Read the model definition and answer for the solid it produces. Units are mm, in the model's axes. Round coordinates to 2 decimals unless told otherwise and drop trailing zeros. Order: outer loops, then holes, each group sorted by start corner. A loop starts at its lowest first (then second) coordinate and runs counter-clockwise, first axis right, second up.
from build123d import *

# Parameters (mm, degrees)
SKETCH1_W           = 96
SKETCH1_H           = 128
BOSS_EXTRUDE1_DEPTH = 2.5
SKETCH2_R           = 1.6
CUT_EXTRUDE1_DEPTH  = 161.019530058
SKETCH3_R           = 1.6
CUT_EXTRUDE2_DEPTH  = 161.019530058
SKETCH4_R           = 1.5
CUT_EXTRUDE3_DEPTH  = 161.019530058
SKETCH9_R           = 1.6
CUT_EXTRUDE4_DEPTH  = 161.019530058
SKETCH12_R          = 3.5
CUT_EXTRUDE5_DEPTH  = 161.019530058
SKETCH13_W          = 23
SKETCH13_H          = 37
SKETCH13_W_2        = 26.25
SKETCH13_H_2        = 57.5
CUT_EXTRUDE6_DEPTH  = 161.019530058


with BuildPart() as part:
    # Sketch1 → Boss-Extrude1 (new body)
    with BuildSketch(Plane.XY):
        with Locations((48, 64)):
            Rectangle(SKETCH1_W, SKETCH1_H)
    extrude(amount=BOSS_EXTRUDE1_DEPTH)

    # Sketch2 → Cut-Extrude1 (cut, through all)
    with BuildSketch(Plane.XY.offset(2.5)):
        with Locations((2, 125)):
            Circle(SKETCH2_R)
        with Locations((27.4, 125)):
            Circle(SKETCH2_R)
        with Locations((78.47, 3)):
            Circle(SKETCH2_R)
        with Locations((68.39, 3)):
            Circle(SKETCH2_R)
        with BuildLine():
            Line((6.15, 126.65), (8.75, 126.65))
            ThreePointArc((8.75, 126.65), (10.4, 125), (8.75, 123.35))
            Line((8.75, 123.35), (6.15, 123.35))
            ThreePointArc((6.15, 123.35), (4.5, 125), (6.15, 126.65))
        make_face()
        with BuildLine():
            Line((87.25, 4.65), (89.85, 4.65))
            ThreePointArc((89.85, 4.65), (91.5, 3), (89.85, 1.35))
            Line((89.85, 1.35), (87.25, 1.35))
            ThreePointArc((87.25, 1.35), (85.6, 3), (87.25, 4.65))
        make_face()
    extrude(amount=-CUT_EXTRUDE1_DEPTH, mode=Mode.SUBTRACT)

    # Sketch3 → Cut-Extrude2 (cut, through all)
    with BuildSketch(Plane.XY.offset(2.5)):
        with Locations((25, 98)):
            Circle(SKETCH3_R)
        with Locations((60, 113)):
            Circle(SKETCH3_R)
        with Locations((25, 29.5)):
            Circle(SKETCH3_R)
    extrude(amount=-CUT_EXTRUDE2_DEPTH, mode=Mode.SUBTRACT)

    # Sketch4 → Cut-Extrude3 (cut, through all)
    with BuildSketch(Plane.XY.offset(2.5)):
        with Locations((13, 15)):
            Circle(SKETCH4_R)
        with Locations((63, 15)):
            Circle(SKETCH4_R)
    extrude(amount=-CUT_EXTRUDE3_DEPTH, mode=Mode.SUBTRACT)

    # Sketch9 → Cut-Extrude4 (cut, through all)
    with BuildSketch(Plane.XY.offset(2.5)):
        with Locations((9, 110.25)):
            Circle(SKETCH9_R)
        with Locations((9, 23.25)):
            Circle(SKETCH9_R)
        with Locations((86, 23.25)):
            Circle(SKETCH9_R)
        with Locations((86, 110.25)):
            Circle(SKETCH9_R)
    extrude(amount=-CUT_EXTRUDE4_DEPTH, mode=Mode.SUBTRACT)

    # Sketch12 → Cut-Extrude5 (cut, through all)
    with BuildSketch(Plane.XY.offset(2.5)):
        with Locations((16.73, 108.25)):
            Circle(SKETCH12_R)
        with Locations((16.73, 93.25)):
            Circle(SKETCH12_R)
        with Locations((16.73, 78.25)):
            Circle(SKETCH12_R)
        with Locations((16.73, 63.25)):
            Circle(SKETCH12_R)
        with Locations((16.73, 48.25)):
            Circle(SKETCH12_R)
        with Locations((16.73, 33.25)):
            Circle(SKETCH12_R)
        with Locations((60, 106.25)):
            Circle(SKETCH12_R)
        with Locations((60, 88.25)):
            Circle(SKETCH12_R)
        with Locations((60, 97.25)):
            Circle(SKETCH12_R)
        with Locations((84.5, 32)):
            Circle(SKETCH12_R)
        with Locations((84.5, 47)):
            Circle(SKETCH12_R)
    extrude(amount=-CUT_EXTRUDE5_DEPTH, mode=Mode.SUBTRACT)

    # Sketch13 → Cut-Extrude6 (cut, through all)
    with BuildSketch(Plane.XY.offset(2.5)):
        with Locations((80.5, 75.75)):
            Rectangle(SKETCH13_W, SKETCH13_H)
        with Locations((46.125, 51.25)):
            Rectangle(SKETCH13_W_2, SKETCH13_H_2)
    extrude(amount=-CUT_EXTRUDE6_DEPTH, mode=Mode.SUBTRACT)


solid = part.part
Q1. A cutting plane is placed at D-D, the plane y = 63.25. Give the vertices of the cut face in (x, z), plus the area to 3 significant figures.
Outcome:
outline: (0, 0) - (13.23, 0) - (13.23, 2.5) - (0, 2.5) - close; (20.23, 0) - (33, 0) - (33, 2.5) - (20.23, 2.5) - close; (59.25, 0) - (69, 0) - (69, 2.5) - (59.25, 2.5) - close; (92, 0) - (96, 0) - (96, 2.5) - (92, 2.5) - close
area: 99.4 mm2
Q2. A flat-ended cylindrical pin translates along its axis: pin 1 (0.8 mm diameter, centred on y = 83, z = 2, fed in from -X). Find the tip coordinate at first contact, or state that the pin passes through.
Outcome:
pin 1: stops at x = 0
Q3. A cutting plane is placed at C-C, the plane x = 38. Give the vertices of the cut face in (y, z), plus the area to 3 significant figures.
Outcome:
outline: (0, 0) - (22.5, 0) - (22.5, 2.5) - (0, 2.5) - close; (80, 0) - (128, 0) - (128, 2.5) - (80, 2.5) - close
area: 176 mm2
Q4. For a pull along X with two mould halves and no side action, classify faces 1 (the face through (96, 63, 1)), 2 (the face through (24.792, 99.586, 1.268)), 3 (the face through (84.4, 110.3, 1.3)), 4 (the face through (47, 0, 1)) as released by +X, released by -X, zero draft, split by the parting line, or undercut.
Outcome:
face 1: released by +X
face 2: undercut
face 3: undercut
face 4: zero draft
Q5. A cutting plane is placed at B-B, the plane x = 78.47. Give the vertices of the cut face in (y, z).
Outcome:
outline: (0, 0) - (1.4, 0) - (1.4, 2.5) - (0, 2.5) - close; (4.6, 0) - (57.25, 0) - (57.25, 2.5) - (4.6, 2.5) - close; (94.25, 0) - (128, 0) - (128, 2.5) - (94.25, 2.5) - close
Q6. A cutting plane is placed at A-A, the plane y = 15. Give the vertices of the cut face in (x, z).
Outcome:
outline: (0, 0) - (11.5, 0) - (11.5, 2.5) - (0, 2.5) - close; (14.5, 0) - (61.5, 0) - (61.5, 2.5) - (14.5, 2.5) - close; (64.5, 0) - (96, 0) - (96, 2.5) - (64.5, 2.5) - close
Q7. Straight lines are drawn through the part: probe 1 along X at (y, z) = (71.5, 1.1); probe 2 along Y at (x, z) = (25, 0.9); probe 3 along X at (y, z) = (26, 0.95). For each, find the intervals that lie inside material, in ascending order.
Outcome:
probe 1: x = 0 to 33, 59.25 to 69, 92 to 96
probe 2: y = 0 to 27.9, 31.1 to 96.4, 99.6 to 128
probe 3: x = 0 to 33, 59.25 to 96
